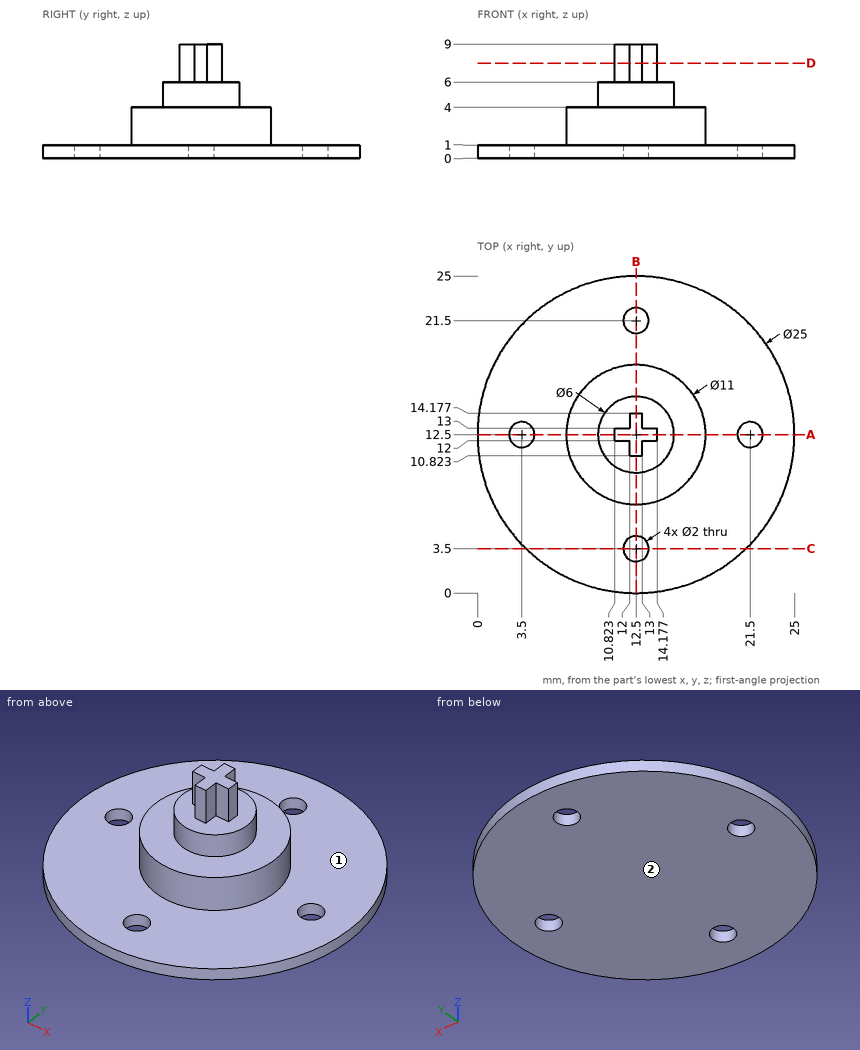
Print and shaded views of the part. All mm, measured from the part's lowest x, y and z. A direction names the side the tool comes from. Round coordinates to 2 decimals unless told otherwise and drop trailing zeros. Order: outer loops, then holes, each group sorted by start corner. A loop starts at its lowest first (then second) coordinate and runs counter-clockwise, first axis right, second up.
Q1. Slice it at D-D (z = 7.5). Write the cut outline in (x, y).
Q2. Drop flat-ended pins along their axis: pin 1 (2 mm diameter, centred on x = 4.5, y = 18.5, fed in from -Z); pin 2 (2.5 mm diameter, centred on x = 12.5, y = 21.5, fed in from +Z); pin 3 (0.8 mm diameter, centred on y = 12.5, z = 7, fed in from -X); pin 4 (0.9 mm diameter, centred on x = 13.5, z = 7.5, fed in from +Y). Give the stop position or say it passes through.
Q3. Which spindle directions (+Z, -Z, +X, -X, +Y, -Y) get a long thin tool onto all of the face, cutting with end or side? Do the marked faces 1 and 2. Say none if no direction does.
Q4. Slice it at C-C (y = 3.5). Write the cut outline in (x, z).
Q5. Slice it at A-A (y = 12.5). Write the cut outline in (x, z), and give its area (3 significant figures).
Q6. Wall check: L1, parallel to Y at x = 12.5, z = 0.65; L2, parallel to Z at x = 18.5, y = 22.25; L3, parallel to X at y = 11.5, z = 8.75. Give the ranges that are in metal, low to high.
Results below:
1. outline: (10.82, 12) - (12, 12) - (12, 10.82) - (13, 10.82) - (13, 12) - (14.18, 12) - (14.18, 13) - (13, 13) - (13, 14.18) - (12, 14.18) - (12, 13) - (10.82, 13) - close
2. pin 1: stops at z = 0
2. pin 2: stops at z = 1
2. pin 3: stops at x = 10.82
2. pin 4: stops at y = 13
3. face 1: +Z
3. face 2: -Z, +X, -X, +Y, -Y
4. outline: (3.83, 0) - (11.5, 0) - (11.5, 1) - (3.83, 1) - close; (13.5, 0) - (21.17, 0) - (21.17, 1) - (13.5, 1) - close
5. outline: (0, 0) - (2.5, 0) - (2.5, 1) - (0, 1) - close; (4.5, 0) - (20.5, 0) - (20.5, 1) - (18, 1) - (18, 4) - (15.5, 4) - (15.5, 6) - (14.18, 6) - (14.18, 9) - (10.82, 9) - (10.82, 6) - (9.5, 6) - (9.5, 4) - (7, 4) - (7, 1) - (4.5, 1) - close; (22.5, 0) - (25, 0) - (25, 1) - (22.5, 1) - close
5. area: 76.1 mm2
6. L1: y = 0 to 2.5, 4.5 to 20.5, 22.5 to 25
6. L2: z = 0 to 1
6. L3: x = 12 to 13
